Input: part model. Units: mm. Frame: model coordinates. A direction names the side the tool comes from. Give positions to 0.01 mm unless a question says otherwise; leave off trailing zeros. Loops run counter-clockwise (first coordinate to the right, second up) from the corner with the lowest first, then second, coordinate; pieces in that order, holes last. Notation, with made-up numbers: (70, 42.25) - (83, 42.25) arc R22 ccw to (83, 51.25) - close; hole circle Ø3 at (-32.75, 61). An arc over 180 degrees is marked (long way). Answer as a JSON object with one key per item and string values. Group by question number.
(1) Pin query (flat end, axial travel): P1, Ø8, axis at x = -347.5, z = -24, coming from the -Y side; P2, Ø2, axis at x = 33, z = -10.5, coming from the +Y side; P3, Ø8, axis at x = 160, y = -19, coming from the +Z side. Return the tip coordinate at first contact, or that it passes through.
(2) Access query for faces 1 (the cylindrical face through (747.856, -30.235, -23.183)), 2 (the flat face through (771.398, -1, 1)), 3 (the cylindrical face through (-747.856, -30.235, -23.183)). Directions: +Z, -Z, +X, -X, +Y, -Y. A direction counts if a zero-diameter tool reaches every point of the face in a straight line with its end or side. Return the directions, or none.
(3) Material intervals for L1, parallel to Z at x = -141, y = 3; L2, parallel to Y at x = 334.5, z = -37.5; L3, parallel to Y at x = 280.5, z = -26, sorted ascending.
(4) Section query B-B (x = 560). Return loops of the section in (y, z) (3 decimals), plus the area to 3 significant figures.
(5) Section query A-A (y = 0). Return loops of the section in (x, z) (3 decimals), plus the area to 3 significant figures.
```python
from build123d import *

# Parameters (mm, degrees)
F0_R       = 53.975
F1_DEPTH   = 590.55
F3_R       = 38.1
F4_DEPTH   = 47.752
F1_FACE_R  = 53.975
F4_FACE_R  = 38.1
F1_FACE1_R = 53.975
F5_FACE_R  = 38.1


with BuildPart() as f1:
    # F0 (on Right) → F1 (new body, symmetric)
    with BuildSketch(Plane.YZ):
        Circle(F0_R)
    extrude(amount=F1_DEPTH, both=True)



with BuildPart() as f4:
    # F3 (on offset) → F4 (new body)
    with BuildSketch(Plane.YZ.offset(771.398)):
        Circle(F3_R)
    extrude(amount=-F4_DEPTH)


with BuildPart() as f5_1:
    # F5: instance of F4
    add(f4.part.mirror(Plane.YZ))


with BuildPart() as f1_1:
    add(f1.part)

    add(f4.part)  # F6 merges F4
    # F1_face (on face) → F6 section 0
    with BuildSketch(Plane.YZ.offset(590.55)):
        Circle(F1_FACE_R)
    # F4_face (on face) → F6 section 1
    with BuildSketch(Plane(origin=(723.646, 0, 0), x_dir=(0, 1, 0), z_dir=(-1, 0, 0))):
        Circle(F4_FACE_R)
    loft()


    add(f5_1.part)  # F7 merges F5_1
    # F1_face1 (on face) → F7 section 0
    with BuildSketch(Plane(origin=(-590.55, 0, 0), x_dir=(0, 1, 0), z_dir=(-1, 0, 0))):
        Circle(F1_FACE1_R)
    # F5_face (on face) → F7 section 1
    with BuildSketch(Plane.YZ.offset(-723.646)):
        Circle(F5_FACE_R)
    loft()


solid = f1_1.part
```
Recorded:
{
 "1": {"P1": "stops at y = -50.13", "P2": "stops at y = 53.13", "P3": "stops at z = 51.85"},
 "2": {"face 1": "+X", "face 2": "+Z, -Z, +X, +Y, -Y", "face 3": "-X"},
 "3": {"L1": "z = -53.89 to 53.89", "L2": "y = -38.82 to 38.82", "L3": "y = -47.3 to 47.3"},
 "4": {"outline": "circle Ø107.95 at (0, 0)", "area": "9,150 mm^2"},
 "5": {"outline": "(-771.398, -38.1) - (-723.646, -38.1) - (-590.55, -53.975) - (590.55, -53.975) - (723.646, -38.1) - (771.398, -38.1) - (771.398, 38.1) - (723.646, 38.1) - (590.55, 53.975) - (-590.55, 53.975) - (-723.646, 38.1) - (-771.398, 38.1) - close", "area": "159,000 mm^2"}
}
